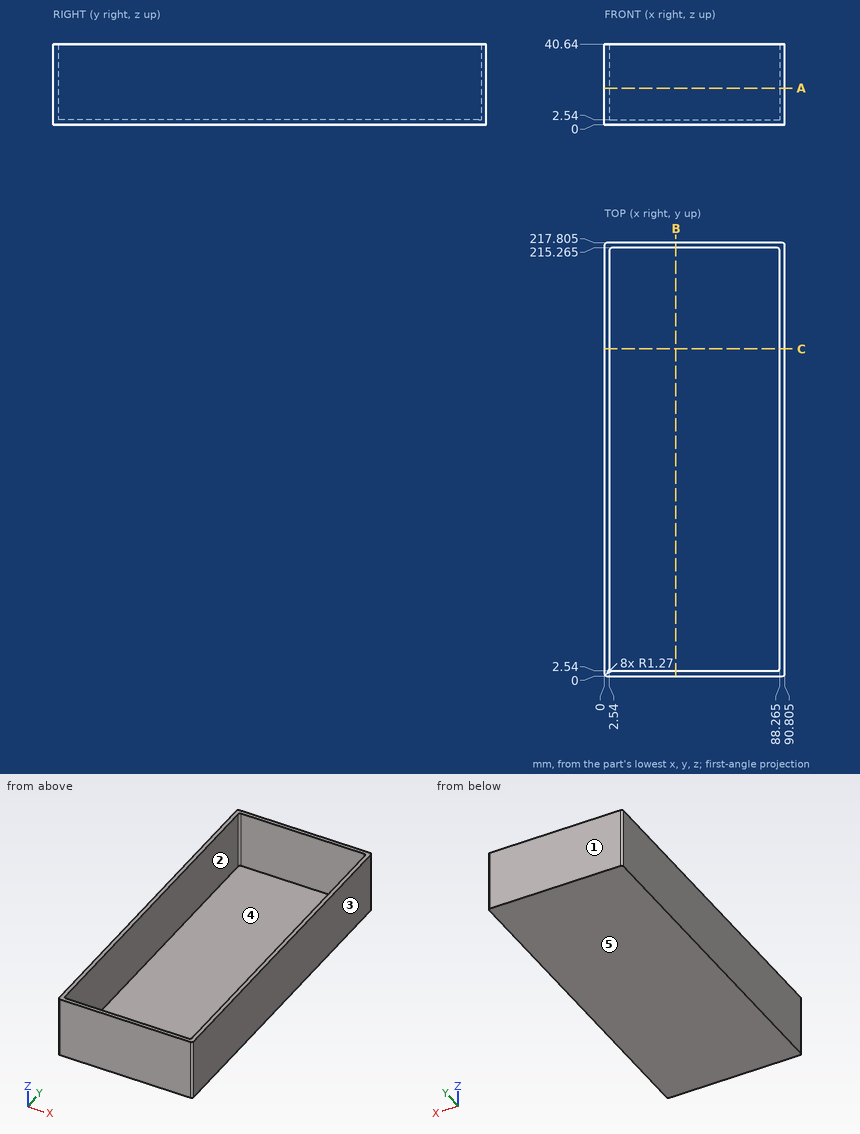
For this review, use the dimensioned drawing (mm, ordinates from the lowest corner) and the shaded views. A direction names the side the tool comes from. Give positions to 0.01 mm unless a question says otherwise; leave off trailing zeros. Order: outer loops, then holes, each group sorted by start corner. A loop starts at its lowest first (then second) coordinate and runs counter-clockwise, first axis right, second up. Notation, with made-up numbers: (1, 43) -> (34, 43) arc R28 ccw to (34, 67) -> close; hole circle Ø1 at (86, 35). An arc over 180 degrees is marked (long way). Write item = value, one per line. Start each with the question number.
(1) Take a section at C-C (y = 164.5). Write out the cut boundary in (x, z) (3 decimals), plus the area to 3 significant figures.
(2) Tool access review of the marked faces 1 and 2: name each direction out of +Z, -Z, +X, -X, +Y, -Y from which nothing blocks a thin tool from reaching the whole face with its end or side.
(3) Draft analysis for pull direction X (two halves, no side actions). For the marked faces 3, 4 and 5, state which applies: +X half, -X half, draft (parallel to the pull), parting line (faces both ways), or undercut.
(4) Take a section at B-B (x = 36). Write out the cut boundary in (y, z) (3 decimals).
(5) For pin 1 Ø6 at (x, y) = (33, 149.5) entering from -Z; pin 2 Ø2 at (x, y) = (10.5, 145.5) entering from +Z, all flat-tipped, find the tip position at first contact; note any pin that passes through.
(6) For L1, parallel to X at y = 62, z = 30.5 (3 decimals); L2, parallel to Y at x = 74.5, z = 5.5 (3 decimals); L3, parallel to Z at x = 75.5, y = 10.5, list the stretches that pass through material, from the lowest coordinate up. Write a range as from..to.
(7) Take a section at A-A (z = 18.5). Write out the cut boundary in (x, y) (3 decimals), plus the area to 3 significant figures.
Returned:
q1.outline = (0, 0) -> (90.805, 0) -> (90.805, 40.64) -> (88.265, 40.64) -> (88.265, 2.54) -> (2.54, 2.54) -> (2.54, 40.64) -> (0, 40.64) -> close
q1.area = 424 mm²
q2.face_1 = +Z, -Z, +X, -X, +Y
q2.face_2 = +Z
q3.face_3 = +X half
q3.face_4 = undercut
q3.face_5 = draft
q4.outline = (0, 0) -> (217.805, 0) -> (217.805, 40.64) -> (215.265, 40.64) -> (215.265, 2.54) -> (2.54, 2.54) -> (2.54, 40.64) -> (0, 40.64) -> close
q5.pin_1 = 0
q5.pin_2 = 2.54
q6.L1 = 0..2.54, 88.265..90.805
q6.L2 = 0..2.54, 215.265..217.805
q6.L3 = 0..2.54
q7.outline = (0, 1.27) arc R1.27 ccw to (1.27, 0) -> (89.535, 0) arc R1.27 ccw to (90.805, 1.27) -> (90.805, 216.535) arc R1.27 ccw to (89.535, 217.805) -> (1.27, 217.805) arc R1.27 ccw to (0, 216.535) -> close; hole (2.54, 3.81) arc R1.27 ccw to (3.81, 2.54) -> (86.995, 2.54) arc R1.27 ccw to (88.265, 3.81) -> (88.265, 213.995) arc R1.27 ccw to (86.995, 215.265) -> (3.81, 215.265) arc R1.27 ccw to (2.54, 213.995) -> close
q7.area = 1,540 mm²
